```python
from build123d import *

# Parameters (mm, degrees)
ESQUISSE1_W                  = 10
ESQUISSE1_H                  = 10
BOSS_EXTRU_1_DEPTH           = 10
ESQUISSE2_R                  = 1.5
ENL_V_MAT_EXTRU_1_DEPTH      = 18.320508076
ESQUISSE3_R                  = 1.5
ENL_V_MAT_EXTRU_2_DEPTH      = 18.320508076
D_GAGEMENT_START             = -1
D_GAGEMENT_M31_OUTLINE_R     = 1.7
D_GAGEMENT_M31_OUTLINE_R_2   = 1.5
D_GAGEMENT_M31_DEPTH         = 12
D_GAGEMENT_M31_2_OUTLINE_R   = 1.7
D_GAGEMENT_M31_2_OUTLINE_R_2 = 1.5
D_GAGEMENT_M31_2_DEPTH       = 12


with BuildPart() as part:
    # Esquisse1 → Boss.-Extru.1 (new body)
    with BuildSketch(Plane.XY):
        with Locations((5, 5)):
            Rectangle(ESQUISSE1_W, ESQUISSE1_H)
    extrude(amount=BOSS_EXTRU_1_DEPTH)

    # Esquisse2 → Enlèv. mat.-Extru.1 (cut, through all)
    with BuildSketch(Plane.XY.offset(10)):
        with Locations((5, 5)):
            Circle(ESQUISSE2_R)
    extrude(amount=-ENL_V_MAT_EXTRU_1_DEPTH, mode=Mode.SUBTRACT)

    # Esquisse3 → Enlèv. mat.-Extru.2 (cut, through all)
    with BuildSketch(Plane.ZY):
        with Locations((5, 5)):
            Circle(ESQUISSE3_R)
    extrude(amount=-ENL_V_MAT_EXTRU_2_DEPTH, mode=Mode.SUBTRACT)

    # Dégagement M31: read off the stored shape, not the designer's step
    # Dégagement M31 outline → Dégagement M31 (cut)
    with BuildSketch(Plane.XY.offset(D_GAGEMENT_START)):
        with Locations((5, 5)):
            Circle(D_GAGEMENT_M31_OUTLINE_R)
        with Locations((5, 5)):
            Circle(D_GAGEMENT_M31_OUTLINE_R_2, mode=Mode.SUBTRACT)
    extrude(amount=D_GAGEMENT_M31_DEPTH, mode=Mode.SUBTRACT)

    # D_gagement M31 2 outline → D_gagement M31 2 (cut)
    with BuildSketch(Plane.YZ.offset(D_GAGEMENT_START)):
        with Locations((5, 5)):
            Circle(D_GAGEMENT_M31_2_OUTLINE_R)
        with Locations((5, 5)):
            Circle(D_GAGEMENT_M31_2_OUTLINE_R_2, mode=Mode.SUBTRACT)
    extrude(amount=D_GAGEMENT_M31_2_DEPTH, mode=Mode.SUBTRACT)


solid = part.part
```
Work out the finished part from the listing and answer in its coordinate system (mm). Coordinates: 2 decimals unless noted, no trailing zeros. Loops run counter-clockwise (first coordinate to the right, second up) from the corner with the lowest first, then second, coordinate; pieces in that order, holes last. Notation, with made-up numbers: M -38.75,-20 L -9.75,-20 A21 cw -9.75,-16 Z; hole C 4,82 d5. An arc over 180 degrees is marked long. Use CSV: the item, a comma, the result in double quotes. Start each with the question number.
(1) Find section B-B, the plane z = 3.5. Give the vertices of the cut face in (x, y).
(2) Find section C-C, the plane x = 1.25. Give the vertices of the cut face in (y, z), then the cut area to 3 significant figures.
(3) Find section D-D, the plane z = 4.75. Give the vertices of the cut face in (x, y), then the cut area to 3 significant figures.
(4) For a pull along Z with two mould halves and no side action, classify faces 1 (the face through (10, 7, 5)), 2 (the face through (8.02, 3.3, 5.07)), 3 (the face through (7, 5, 10)) as +Z half, -Z half, draft (parallel to the pull), parting line (faces both ways), or undercut.
(5) Find section A-A, the plane y = 5. Give the vertices of the cut face in (x, z), then the cut area to 3 significant figures.
(6) Consider line 1 (X direction, y = 5, z = 1.8). Determine where the line is inside the solid, lowest interval first.
Recorded:
1,outline,"M 0,0 L 10,0 L 10,4.2 L 6.5,4.2 A1.7 cw 3.5,4.2 L 0,4.2 Z; M 0,5.8 L 3.5,5.8 A1.7 cw 6.5,5.8 L 10,5.8 L 10,10 L 0,10 Z"
2,outline,"M 0,0 L 10,0 L 10,10 L 0,10 Z; hole C 5,5 d3.4"
2,area,"90.9 mm^2"
3,outline,"M 0,0 L 10,0 L 10,3.32 L 5.25,3.32 A1.7 cw 4.75,3.32 L 0,3.32 Z; M 0,6.68 L 4.75,6.68 A1.7 cw 5.25,6.68 L 10,6.68 L 10,10 L 0,10 Z"
3,area,"66.4 mm^2"
4,face 1,"draft"
4,face 2,"undercut"
4,face 3,"+Z half"
5,outline,"M 0,0 L 3.3,0 L 3.3,3.3 L 0,3.3 Z; M 0,6.7 L 3.3,6.7 L 3.3,10 L 0,10 Z; M 6.7,0 L 10,0 L 10,3.3 L 6.7,3.3 Z; M 6.7,6.7 L 10,6.7 L 10,10 L 6.7,10 Z"
5,area,"43.6 mm^2"
6,line 1,"x = 0 to 3.3, 6.7 to 10"
